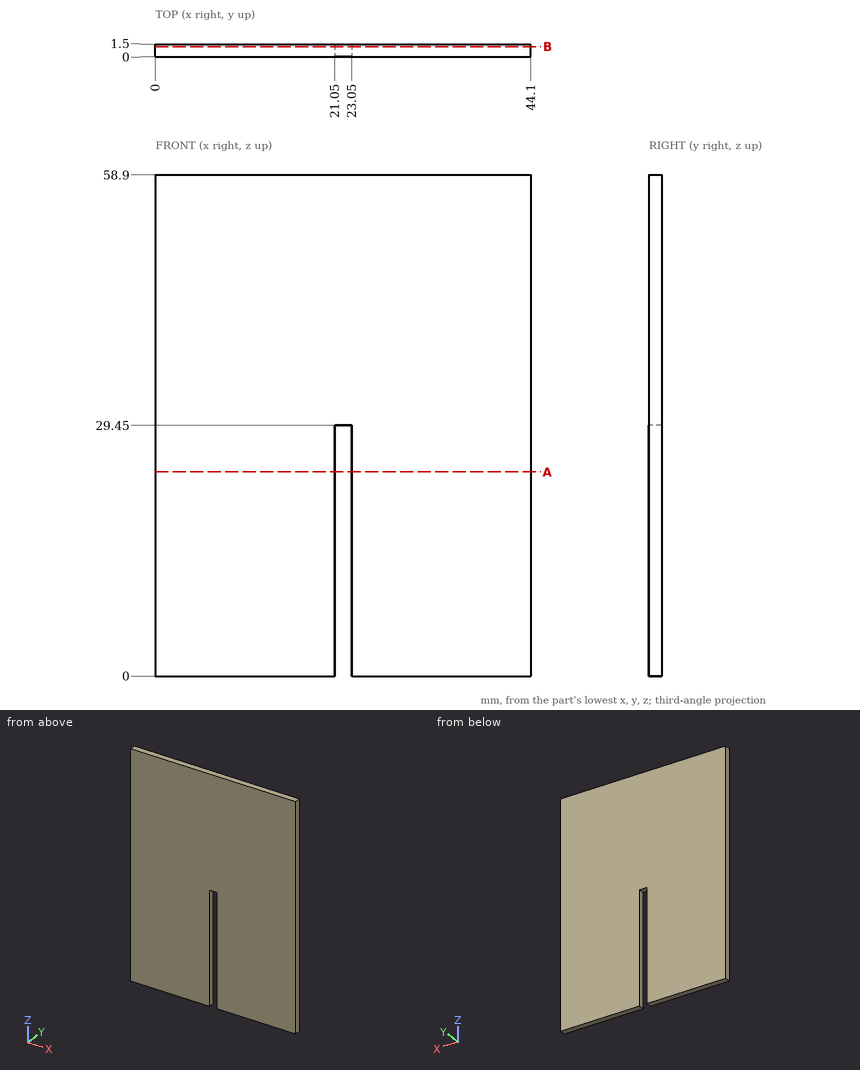
Geometry: see drawing. Coordinates: mm, zero at the bounding-box minimum. Coordinates: 2 decimals unless noted, no trailing zeros. Order: outer loops, then holes, each group sorted by start corner. A loop starts at its lowest first (then second) coordinate and runs counter-clockwise, first axis right, second up. Notation, with made-up numbers: (66.25, 62) - (123.25, 62) arc R26 cw to (123.25, 82) - close; hole circle Ø5 at (-12, 69). An arc over 180 degrees is marked (long way). Use one line per item in the form item = value.
1) Ray query, L1, parallel to X at y = 1.2, z = 13; L2, parallel to Z at x = 23, y = 0.1. Return the intervals inside material, ascending.
Solutions:
L1 = 0 to 21.05, 23.05 to 44.1
L2 = 29.45 to 58.9
2) Section A-A (z = 24). Return loops of the section in (x, y).
Solutions:
outline = (0, 0) - (21.05, 0) - (21.05, 1.5) - (0, 1.5) - close; (23.05, 0) - (44.1, 0) - (44.1, 1.5) - (23.05, 1.5) - close
3) Section B-B (y = 1.2). Return loops of the section in (x, z).
Solutions:
outline = (0, 0) - (21.05, 0) - (21.05, 29.45) - (23.05, 29.45) - (23.05, 0) - (44.1, 0) - (44.1, 58.9) - (0, 58.9) - close
4) Pin query (flat end, axial travel): pin 1 (0.8 mm diameter, centred on x = 22.5, y = 1, fed in from -Z). Return the tip coordinate at first contact, or that it passes through.
Solutions:
pin_1 = 29.45
